Work out the finished part from the listing and answer in its coordinate system (mm). Face numbers are marked on the shaded views. A direction names the side the tool comes from. Round coordinates to 2 decimals unless told otherwise and drop trailing zeros. Loops run counter-clockwise (first coordinate to the right, second up) from the corner with the lowest first, then second, coordinate; pieces in that order, holes last. Notation, with made-up numbers: (27.5, -22.5) - (83.5, -22.5) arc R27 cw to (83.5, -6.5) - close; hole circle Ø7 at (-17, 57.25). An arc over 180 degrees is marked (long way). Return JSON: item names as keys, results as strings.
from build123d import *

# Parameters (mm, degrees)
SCHIZZO1_W                   = 50
SCHIZZO1_H                   = 50
SCHIZZO1_R                   = 17.5
ESTRUSIONE_ESTRUSIONE1_DEPTH = 12
SCHIZZO2_R                   = 2.5
TAGLIO_ESTRUSIONE1_DEPTH     = 5
SCHIZZO3_R                   = 2.5
TAGLIO_ESTRUSIONE2_DEPTH     = 5


with BuildPart() as part:
    # Schizzo1 → Estrusione-Estrusione1 (new body)
    with BuildSketch(Plane.XY):
        Rectangle(SCHIZZO1_W, SCHIZZO1_H)
        Circle(SCHIZZO1_R, mode=Mode.SUBTRACT)
    extrude(amount=ESTRUSIONE_ESTRUSIONE1_DEPTH)

    # Schizzo2 → Taglio-Estrusione1 (cut)
    with BuildSketch(Plane(origin=(0, -25, 0), x_dir=(-1, 0, 0), z_dir=(0, -1, 0))):
        with Locations((21, -6)):
            Circle(SCHIZZO2_R)
        with Locations((-20, -6)):
            Circle(SCHIZZO2_R)
    extrude(amount=-TAGLIO_ESTRUSIONE1_DEPTH, mode=Mode.SUBTRACT)

    # Schizzo3 → Taglio-Estrusione2 (cut)
    with BuildSketch(Plane(origin=(0, 25, 0), x_dir=(1, 0, 0), z_dir=(0, 1, 0))):
        with Locations((20, -6)):
            Circle(SCHIZZO3_R)
        with Locations((-21, -6)):
            Circle(SCHIZZO3_R)
    extrude(amount=-TAGLIO_ESTRUSIONE2_DEPTH, mode=Mode.SUBTRACT)


solid = part.part
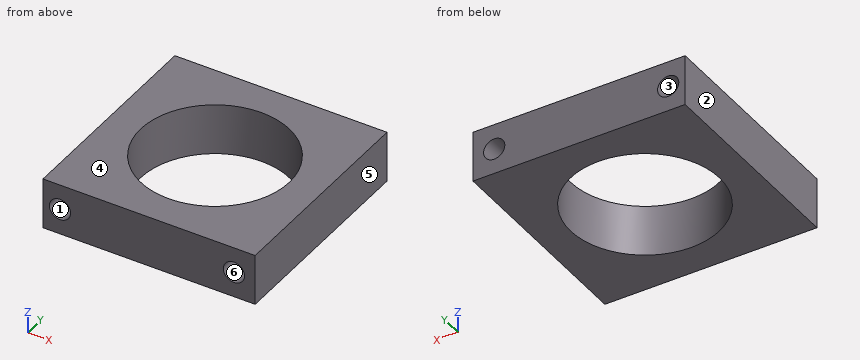
1) Flat-ended cylindrical pins translate along their axes: pin 1 (4 mm diameter, centred on x = 20, z = 6, fed in from +Y); pin 2 (4 mm diameter, centred on x = 19, z = 5.5, fed in from +Y); pin 3 (2.5 mm diameter, centred on x = -20, z = 5.5, fed in from -Y). Find the tip coordinate at first contact, or state that the pin passes through.
Verdict:
{"pin 1": "stops at y = 20", "pin 2": "stops at y = 25", "pin 3": "stops at y = -20"}
2) A tool of negligible diameter and unlimited length cuts with its end or side. For the marked faces 1, 2 and 3, from which of +Z, -Z, +X, -X, +Y, -Y can it reach the whole face along a straight path? Write none if from no direction.
Verdict:
{"face 1": "-Y", "face 2": "+Z, -Z, -X, +Y, -Y", "face 3": "+Y"}
3) Section B-B (z = 2.5) is taken. Give the vertices of the cut face in (x, y).
Verdict:
{"outline": "(-25, -25) - (25, -25) - (25, 25) - (-25, 25) - close; hole circle Ø35 at (0, 0)"}
4) Determine the mould class of the marked faces 4, 5 and 6 for opening direction X: pulls with the +X half, pulls with the -X half, needs draft (parallel to the pull), parting line crosses it, or undercut.
Verdict:
{"face 4": "needs draft", "face 5": "pulls with the +X half", "face 6": "undercut"}
5) Find the intervals of material crossed by L1, parallel to X at y = 22.25, z = 6; L2, parallel to Z at x = 20, y = -22; L3, parallel to Y at x = 0, z = 8.5, in increasing order.
Verdict:
{"L1": "x = -25 to -23.5, -18.5 to 17.5, 22.5 to 25", "L2": "z = 0 to 3.5, 8.5 to 12", "L3": "y = -25 to -17.5, 17.5 to 25"}
6) Section A-A (x = 10.5) is taken. Give the vertices of the cut face in (y, z), and give its area (3 significant figures).
Verdict:
{"outline": "(-25, 0) - (-14, 0) - (-14, 12) - (-25, 12) - close; (14, 0) - (25, 0) - (25, 12) - (14, 12) - close", "area": "264 mm2"}
7) Section C-C (y = 0) is taken. Give the vertices of the cut face in (x, z).
Verdict:
{"outline": "(-25, 0) - (-17.5, 0) - (-17.5, 12) - (-25, 12) - close; (17.5, 0) - (25, 0) - (25, 12) - (17.5, 12) - close"}
8) Section D-D (x = -21) is taken. Give the vertices of the cut face in (y, z), and give its area (3 significant figures).
Verdict:
{"outline": "(-25, 0) - (25, 0) - (25, 3.5) - (20, 3.5) - (20, 8.5) - (25, 8.5) - (25, 12) - (-25, 12) - (-25, 8.5) - (-20, 8.5) - (-20, 3.5) - (-25, 3.5) - close", "area": "550 mm2"}
